```python
from build123d import *

# Parameters (mm, degrees)
F1_DEPTH = 25
F2_R     = 4.99999
F3_R     = 4.99999


# Not quite as in the source:
# - a fillet or chamfer is up to 0.001 mm smaller than in the source, because OpenCascade refuses the exact size


with BuildPart() as f1:
    # F0 (on Top) → F1 (new body)
    with BuildSketch(Plane.XY):
        with BuildLine():
            Line((-16, 0), (-11, 0))
            Line((-11, 0), (-11, 15))
            ThreePointArc((-11, 15), (-9.5355339059, 18.5355339059), (-6, 20))
            Line((-6, 20), (-5, 20))
            ThreePointArc((-5, 20), (-1.4644660941, 18.5355339059), (0, 15))
            Line((0, 15), (0, -20))
            Line((0, -20), (20, -20))
            ThreePointArc((20, -20), (27.0710678119, -17.0710678119), (30, -10))
            Line((30, -10), (30, 10))
            Line((30, 10), (25, 10))
            Line((25, 10), (25, -1.100000754))
            Line((25, -1.100000754), (25, -5))
            ThreePointArc((25, -5), (22.0710678119, -12.0710678119), (15, -15))
            ThreePointArc((15, -15), (7.9289321881, -12.0710678119), (5, -5))
            Line((5, -5), (5, 15))
            ThreePointArc((5, 15), (2.0710678119, 22.0710678119), (-5, 25))
            Line((-5, 25), (-6, 25))
            ThreePointArc((-6, 25), (-13.0710678119, 22.0710678119), (-16, 15))
            Line((-16, 15), (-16, 0))
        make_face()
    extrude(amount=F1_DEPTH)

    # F2 (radius 5 in the source; OpenCascade refuses exactly that, so slightly less here)
    f2_edges = [f1.edges().sort_by_distance(p)[0] for p in [
        (30, 10, 12.5),
    ]]
    fillet(f2_edges, radius=F2_R)

    # F3 (radius 5 in the source; OpenCascade refuses exactly that, so slightly less here)
    f3_edges = [f1.edges().sort_by_distance(p)[0] for p in [
        (-16, 0, 12.5),
    ]]
    fillet(f3_edges, radius=F3_R)


solid = f1.part
```
Model file for the job. Use its own axes, mm. A direction names the side the tool comes from. Coordinates: 2 decimals unless noted, no trailing zeros. Loops run counter-clockwise (first coordinate to the right, second up) from the corner with the lowest first, then second, coordinate; pieces in that order, holes last. Notation, with made-up numbers: (56, 2.25) - (108, 2.25) arc R16 ccw to (108, 23.25) - close; hole circle Ø5 at (14.25, 8). An arc over 180 degrees is marked (long way). Write item = value, one per line. Start each with the question number.
Item 1: Saw through at A-A, the plane y = 12. List the corners of the cut face in (x, z), then the cut area to 3 significant figures.
Item 2: Saw through at D-D, the plane y = -8. List the corners of the cut face in (x, z).
Item 3: Pull direction X, two halves, no side cores. Call faces 1 (the face through (26.99, -17.15, 12.32)), 2 (the face through (25, 3, 12)), 3 (the face through (-14, 1, 13)): +X half, -X half, draft (parallel to the pull), parting line (faces both ways), or undercut.
Item 4: Drop flat-ended pins along their axis: pin 1 Ø7.5 at (y, z) = (-2, 17.5) entering from -X; pin 2 Ø5 at (y, z) = (11, 5.5) entering from +X; pin 3 Ø2 at (y, z) = (1.5, 16.5) entering from -X. Give the stop position or say it passes through.
Item 5: 3-axis set-ups, long thin cutter, end or side, ignore diameter. For faces 4 (the face through (-16, 10, 12)), 5 (the face through (5, 5, 12)), 6 (the face through (-10, 18, 12)): which of +Z, -Z, +X, -X, +Y, -Y reach the whole face in a straight line?
Item 6: Saw through at B-B, the plane y = 1. List the corners of the cut face in (x, z), then the cut area to 3 significant figures.
Item 7: Wall check: probe 1 along X at (y, z) = (-1.5, 16.25); probe 2 along X at (y, z) = (4.5, 8); probe 3 along X at (y, z) = (6.5, 3.5). Give the ranges that are in metal, low to high. Write a range as [from, to].
Answers:
q1.outline = (-16, 0) - (-11, 0) - (-11, 25) - (-16, 25) - close; (0, 0) - (5, 0) - (5, 25) - (0, 25) - close
q1.area = 250 mm2
q2.outline = (0, 0) - (5.46, 0) - (5.46, 25) - (0, 25) - close; (24.54, 0) - (30, 0) - (30, 25) - (24.54, 25) - close
q3.face_1 = +X half
q3.face_2 = undercut
q3.face_3 = -X half
q4.pin_1 = -14.8
q4.pin_2 = 28.57
q4.pin_3 = -15.33
q5.face_4 = +Z, -Z, -X, +Y, -Y
q5.face_5 = +Z, -Z, +Y
q5.face_6 = +Z, -Z, -Y
q6.outline = (-14, 0) - (-11, 0) - (-11, 25) - (-14, 25) - close; (0, 0) - (5, 0) - (5, 25) - (0, 25) - close; (25, 0) - (30, 0) - (30, 25) - (25, 25) - close
q6.area = 325 mm2
q7.probe_1 = [0, 5], [25, 30]
q7.probe_2 = [-15.97, -11], [0, 5], [25, 30]
q7.probe_3 = [-16, -11], [0, 5], [25, 29.77]
